The model under review builds one solid part; all positions refer to its coordinate system, in mm. Give positions to 0.01 mm unless a question says otherwise; leave off trailing zeros. Write each loop counter-clockwise with the first axis right and the second up, starting at its lowest first coordinate (ties: lowest second). Pieces come first, ordered by that corner, then holes.
from build123d import *

# Parameters (mm, degrees)
BOSS_EXTRUDE1_DEPTH = 9
SKETCH2_R           = 2.25
CUT_EXTRUDE1_DEPTH  = 229.5
FILLET1_R           = 2
SKETCH3_R           = 4.5
SKETCH3_R_2         = 2.5
BOSS_EXTRUDE2_DEPTH = 10


with BuildPart() as part:
    # Sketch1 → Boss-Extrude1 (new body)
    with BuildSketch(Plane.XY):
        Polygon((-110.25, 0), (110.25, 0), (110.25, -38), (114.25, -38), (114.25, 4), (-114.25, 4), (-114.25, -38), (-110.25, -38), align=None)
    extrude(amount=BOSS_EXTRUDE1_DEPTH)

    # Sketch2 → Cut-Extrude1 (cut, through all)
    with BuildSketch(Plane(origin=(114.25, 0, 0), x_dir=(0, 0, -1), z_dir=(1, 0, 0))):
        with Locations((-4.5, -13.5)):
            Circle(SKETCH2_R)
        with BuildLine():
            ThreePointArc((-4.5, -38), (-7.681980515, -36.681980515), (-9, -33.5))
            Line((-9, -33.5), (-9, -38))
            Line((-9, -38), (-4.5, -38))
        make_face()
        with BuildLine():
            Line((0, -38), (0, -33.5))
            ThreePointArc((0, -33.5), (-1.318019485, -36.681980515), (-4.5, -38))
            Line((-4.5, -38), (0, -38))
        make_face()
        with Locations((-4.5, -33.5)):
            Circle(SKETCH2_R)
    extrude(amount=-CUT_EXTRUDE1_DEPTH, mode=Mode.SUBTRACT)

    # Fillet1
    fillet1_edges = [part.edges().sort_by_distance(p)[0] for p in [
        (114.25, 4, 4.5),
        (-114.25, 4, 4.5),
    ]]
    fillet(fillet1_edges, radius=FILLET1_R)

    # Sketch3 → Boss-Extrude2 (add)
    with BuildSketch(Plane(origin=(0, 4, 0), x_dir=(1, 0, 0), z_dir=(0, 1, 0))):
        with Locations((0, -4.5)):
            Circle(SKETCH3_R)
        with Locations((0, -4.5)):
            Circle(SKETCH3_R_2, mode=Mode.SUBTRACT)
        with Locations((60, -4.5)):
            Circle(SKETCH3_R)
        with Locations((60, -4.5)):
            Circle(SKETCH3_R_2, mode=Mode.SUBTRACT)
        with Locations((-60, -4.5)):
            Circle(SKETCH3_R)
        with Locations((-60, -4.5)):
            Circle(SKETCH3_R_2, mode=Mode.SUBTRACT)
    extrude(amount=BOSS_EXTRUDE2_DEPTH)


solid = part.part
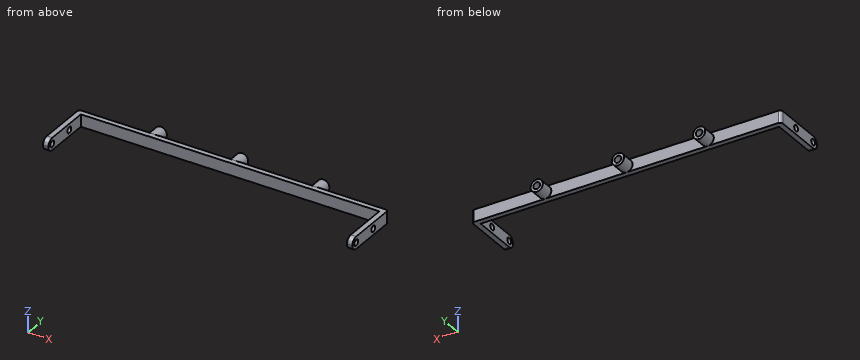
1) Insertion check: pin 1 (3 mm diameter, centred on x = -16, z = 7, fed in from -Y); pin 2 (4 mm diameter, centred on x = -27.5, z = 2.5, fed in from +Y). Each pin has a flat end and moves straight along its axis. Give the tip position at first contact, or say it passes through.
2) To check wall thickness, follow probe 1 along Y at (x, z) = (-112, 4.5); probe 2 along X at (y, z) = (-18, 8.75); probe 3 along Y at (x, z) = (113.45, 4.5). State the ranges of each line that lie inside material, in increasing order.
3) Consider section B-B, the plane x = 24. Give the boundary of the cut face in (y, z), then the cut area to 3 significant figures.
4) Consider section A-A, the plane y = -13.5. Give the boundary of the cut face in (x, z).
Answer block:
1. pin 1: stops at y = 0
1. pin 2: stops at y = 4
2. probe 1: y = -38 to -35.75, -31.25 to -15.75, -11.25 to 4
2. probe 2: x = -114.25 to -110.25, 110.25 to 114.25
2. probe 3: y = -38 to -35.75, -31.25 to -15.75, -11.25 to 3.6
3. outline: (0, 0) - (4, 0) - (4, 9) - (0, 9) - close
3. area: 36.0 mm2
4. outline: (-114.25, 0) - (-110.25, 0) - (-110.25, 2.25) - (-114.25, 2.25) - close; (-114.25, 6.75) - (-110.25, 6.75) - (-110.25, 9) - (-114.25, 9) - close; (110.25, 0) - (114.25, 0) - (114.25, 2.25) - (110.25, 2.25) - close; (110.25, 6.75) - (114.25, 6.75) - (114.25, 9) - (110.25, 9) - close
